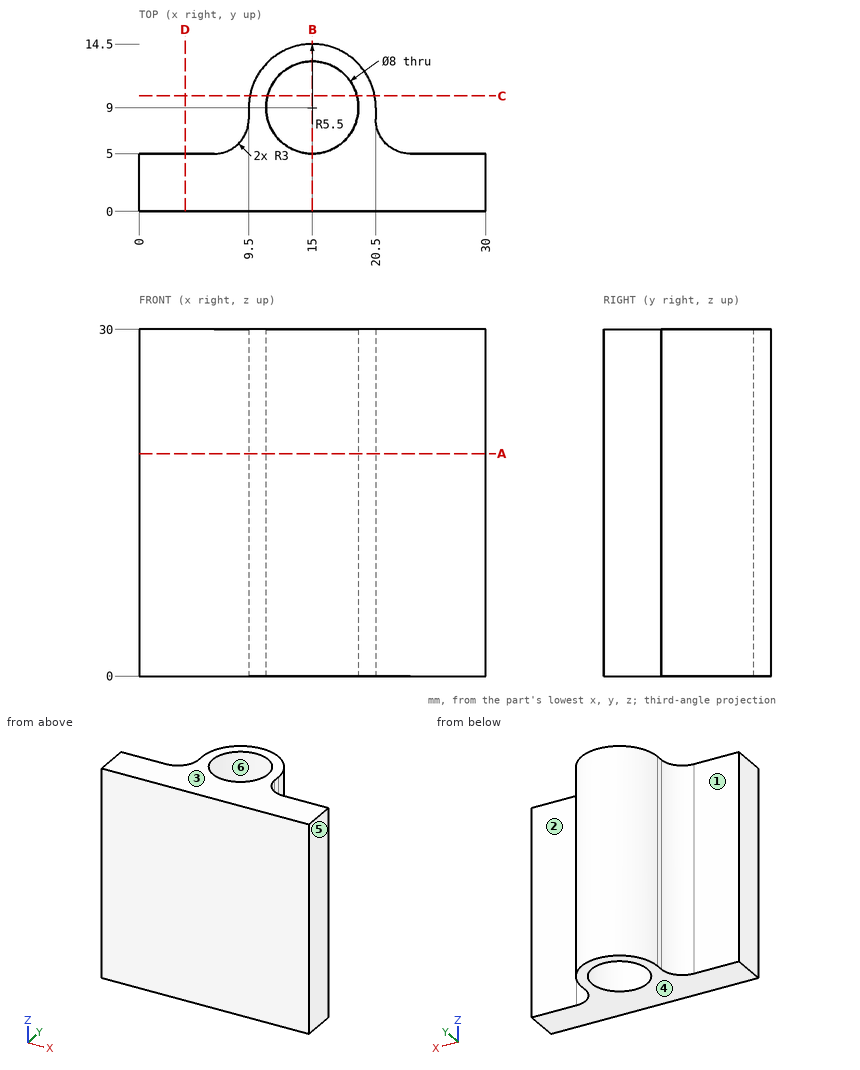
Drawing for the job (mm, zero at the part's lowest x, y, z). A direction names the side the tool comes from. Give positions to 0.01 mm unless a question says otherwise; leave off trailing zeros. Order: outer loops, then holes, each group sorted by start corner. A loop starts at its lowest first (then second) coordinate and runs counter-clockwise, first axis right, second up. Notation, with made-up numbers: (55, 3.25) - (80, 3.25) arc R29 ccw to (80, 33.25) - close; hole circle Ø4 at (86.5, 42.25). An arc over 180 degrees is marked (long way). Use one line per item in the form item = value.
Item 1: Which spindle directions (+Z, -Z, +X, -X, +Y, -Y) get a long thin tool onto all of the face, cutting with end or side? Do the marked faces 1, 2 and 3. Say none if no direction does.
Solution:
face_1 = +Z, -Z, -X, +Y
face_2 = +Z, -Z, +X, +Y
face_3 = +Z, +X, -X, +Y, -Y
Item 2: Two-plate mould, pull along X, no slides. Class the marked faces 4, 5 and 6: released by +X, released by -X, zero draft, split by the parting line, or undercut.
Solution:
face_4 = zero draft
face_5 = released by +X
face_6 = undercut
Item 3: Pin check, flat tips, straight feed: pin 1 Ø0.5 at (y, z) = (8.5, 14.5) entering from +X; pin 2 Ø1.5 at (x, z) = (23.5, 14.5) entering from +Y; pin 3 Ø1 at (x, z) = (3, 8.5) entering from +Y. Stop position of each tip, or through.
Solution:
pin_1 = 20.5
pin_2 = 5.1
pin_3 = 5
Item 4: Probe probe 1 along X at (y, z) = (9, 16.5); probe 2 along Y at (x, z) = (15, 9); probe 3 along Y at (x, z) = (4.5, 13.25). List the from-to ranges inside material, lowest first. Write a range as from..to.
Solution:
probe_1 = 9.5..11, 19..20.5
probe_2 = 0..5, 13..14.5
probe_3 = 0..5
Item 5: Slice it at C-C on y = 10. Give the cut face in (x, z).
Solution:
outline = (9.59, 0) - (11.13, 0) - (11.13, 30) - (9.59, 30) - close; (18.87, 0) - (20.41, 0) - (20.41, 30) - (18.87, 30) - close
Item 6: Slice it at B-B on x = 15. Give the cut face in (y, z).
Solution:
outline = (0, 0) - (5, 0) - (5, 30) - (0, 30) - close; (13, 0) - (14.5, 0) - (14.5, 30) - (13, 30) - close
Item 7: Slice it at A-A on z = 19.25. Give the cut face in (x, y).
Solution:
outline = (0, 0) - (30, 0) - (30, 5) - (23.5, 5) arc R3 cw to (20.5, 8) - (20.5, 9) arc R5.5 ccw to (9.5, 9) - (9.5, 8) arc R3 cw to (6.5, 5) - (0, 5) - close; hole circle Ø8 at (15, 9)
Item 8: Slice it at D-D on x = 4. Give the cut face in (y, z), and give its area (3 significant figures).
Solution:
outline = (0, 0) - (5, 0) - (5, 30) - (0, 30) - close
area = 150 mm2
